Geometry: see drawing. Coordinates: mm, zero at the bounding-box minimum. A direction names the side the tool comes from. Coordinates: 2 decimals unless noted, no trailing zeros. Write each loop counter-clockwise with the first axis right and the second up, starting at its lowest first coordinate (ties: lowest second). Pieces come first, ordered by that corner, then holes. Notation, with made-up numbers: M -40,35.5 L -20,35.5 A17 ccw -20,40.5 Z; hole C -26,61 d3. An arc over 180 degrees is marked long. One line per item, written item: value. Start each with the question number.
Item 1: Mould query, pull axis Y, two halves, no side actions, for the marked faces 1, 2, 3 and 4. Classes: released by +Y, released by -Y, zero draft, split by the parting line, or undercut.
Item 2: Ray query, L1, parallel to Y at x = 33, z = 56.5 (1 decimal); L2, parallel to X at y = 12, z = 51; L3, parallel to Y at x = 3, z = 7.5 (1 decimal). Return the intervals inside material, ascending. Write a range as from..to.
Item 3: Cut plane B-B, the plane y = 10. Output: boundary loops of the cut face in (x, z) (1 decimal).
Item 4: Cut plane C-C, the plane z = 75. Output: boundary loops of the cut face in (x, y) (1 decimal).
Item 5: Cut plane A-A, the plane x = 29. Output: boundary loops of the cut face in (y, z) (1 decimal).
Item 6: Pin query (flat end, axial travel): P1, Ø6, axis at y = 14, z = 62, coming from the -X side. Return the tip coordinate at first contact, or that it passes through.
Item 7: Set-up query: the marked faces 5 and 6. Return all of +Z, -Z, +X, -X, +Y, -Y with unobstructed straight access to the full face (end or side cutting, diameter ignored); none if empty.
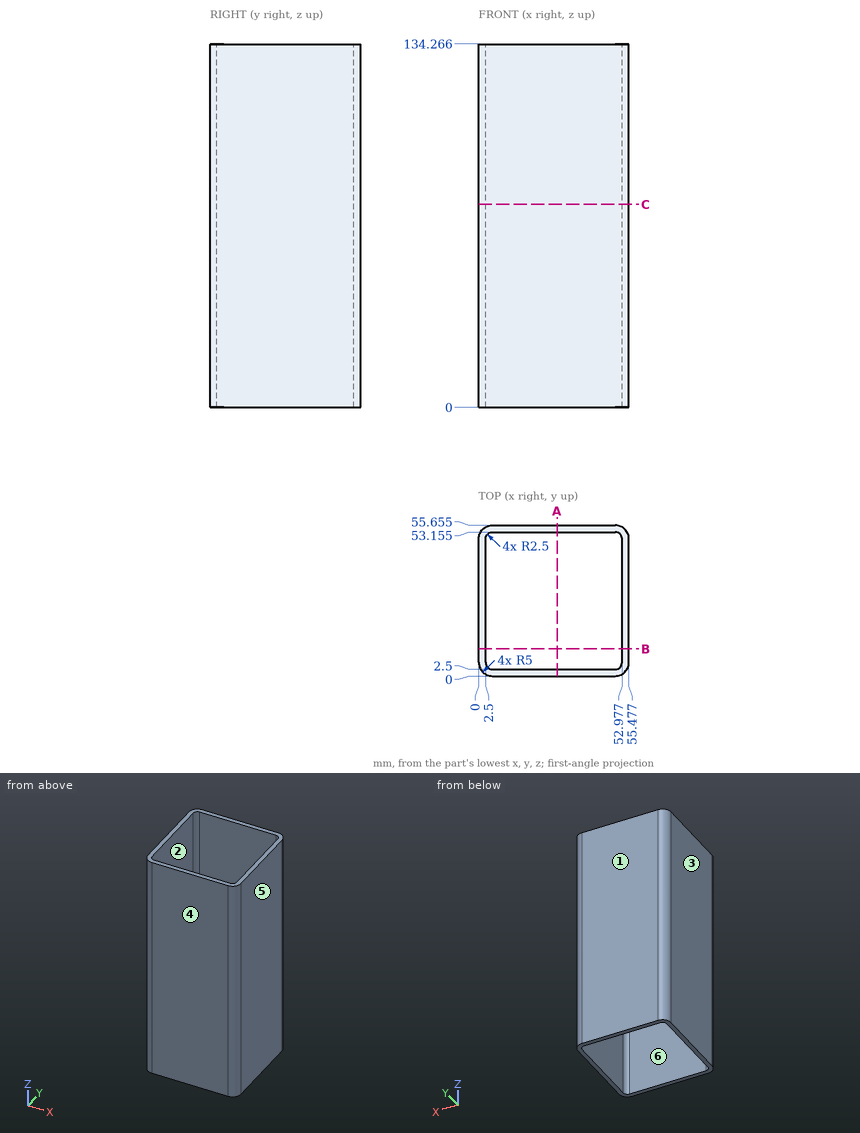
From the geometry:
1. face 1: released by +Y
1. face 2: undercut
1. face 3: zero draft
1. face 4: released by -Y
2. L1: y = 0..2.5, 53.2..55.7
2. L2: x = 0..2.5, 52.98..55.48
2. L3: y = 0.4..3.5, 52.2..55.2
3. outline: M 0,0 L 2.5,0 L 2.5,134.3 L 0,134.3 Z; M 53,0 L 55.5,0 L 55.5,134.3 L 53,134.3 Z
4. outline: M 0,5 A5 ccw 5,0 L 50.5,0 A5 ccw 55.5,5 L 55.5,50.7 A5 ccw 50.5,55.7 L 5,55.7 A5 ccw 0,50.7 Z; hole M 2.5,5 A2.5 ccw 5,2.5 L 50.5,2.5 A2.5 ccw 53,5 L 53,50.7 A2.5 ccw 50.5,53.2 L 5,53.2 A2.5 ccw 2.5,50.7 Z
5. outline: M 0,0 L 2.5,0 L 2.5,134.3 L 0,134.3 Z; M 53.2,0 L 55.7,0 L 55.7,134.3 L 53.2,134.3 Z
6. P1: stops at x = 0
7. face 5: +Z, -Z, +X, +Y, -Y
7. face 6: +Z, -Z
